```python
from build123d import *

# Parameters (mm, degrees)
SKETCH_2_W          = 9
SKETCH_2_H          = 6.5
EXTRUDE_1_DEPTH     = 90
SKETCH_3_R          = 3
CUT_EXTRUDE_1_DEPTH = 3.5
SKETCH_4_R          = 1.75
CUT_EXTRUDE_2_DEPTH = 91.346554998


with BuildPart() as part:
    # 草图2 → 凸台-拉伸1 (new body)
    with BuildSketch(Plane(origin=(0, 0, 0), x_dir=(0, 0, -1), z_dir=(1, 0, 0))):
        Rectangle(SKETCH_2_W, SKETCH_2_H)
    extrude(amount=EXTRUDE_1_DEPTH)

    # 草图3 → 切除-拉伸1 (cut)
    with BuildSketch(Plane(origin=(0, 3.25, 0), x_dir=(1, 0, 0), z_dir=(0, 1, 0))):
        with Locations(Location((15, 0, 0), (0, 0, 270))):
            Circle(SKETCH_3_R)
        with Locations(Location((35, 0, 0), (0, 0, 270))):
            Circle(SKETCH_3_R)
        with Locations(Location((55, 0, 0), (0, 0, 270))):
            Circle(SKETCH_3_R)
        with Locations(Location((75, 0, 0), (0, 0, 270))):
            Circle(SKETCH_3_R)
        with Locations((95, 0)):
            Circle(SKETCH_3_R)
        with Locations((115, 0)):
            Circle(SKETCH_3_R)
        with Locations((135, 0)):
            Circle(SKETCH_3_R)
        with Locations((155, 0)):
            Circle(SKETCH_3_R)
        with Locations((175, 0)):
            Circle(SKETCH_3_R)
        with Locations((195, 0)):
            Circle(SKETCH_3_R)
        with Locations((215, 0)):
            Circle(SKETCH_3_R)
        with Locations((235, 0)):
            Circle(SKETCH_3_R)
        with Locations((255, 0)):
            Circle(SKETCH_3_R)
    extrude(amount=-CUT_EXTRUDE_1_DEPTH, mode=Mode.SUBTRACT)

    # 草图4 → 切除-拉伸2 (cut, through all)
    with BuildSketch(Plane(origin=(0, 3.25, 0), x_dir=(1, 0, 0), z_dir=(0, 1, 0))):
        with Locations(Location((15, 0, 0), (0, 0, 270))):
            Circle(SKETCH_4_R)
        with Locations(Location((35, 0, 0), (0, 0, 270))):
            Circle(SKETCH_4_R)
        with Locations(Location((55, 0, 0), (0, 0, 270))):
            Circle(SKETCH_4_R)
        with Locations(Location((75, 0, 0), (0, 0, 270))):
            Circle(SKETCH_4_R)
        with Locations((95, 0)):
            Circle(SKETCH_4_R)
        with Locations((115, 0)):
            Circle(SKETCH_4_R)
        with Locations((135, 0)):
            Circle(SKETCH_4_R)
        with Locations((155, 0)):
            Circle(SKETCH_4_R)
        with Locations((175, 0)):
            Circle(SKETCH_4_R)
        with Locations((195, 0)):
            Circle(SKETCH_4_R)
        with Locations((215, 0)):
            Circle(SKETCH_4_R)
        with Locations((235, 0)):
            Circle(SKETCH_4_R)
        with Locations((255, 0)):
            Circle(SKETCH_4_R)
    extrude(amount=-CUT_EXTRUDE_2_DEPTH, mode=Mode.SUBTRACT)


solid = part.part
```
Geometry: final body of the model. Coordinates: model frame, mm. A direction names the side the tool comes from. Coordinates: 2 decimals unless noted, no trailing zeros. Order: outer loops, then holes, each group sorted by start corner. A loop starts at its lowest first (then second) coordinate and runs counter-clockwise, first axis right, second up. Notation, with made-up numbers: (37, 83) - (61, 83) arc R19 cw to (61, 112) - close; hole circle Ø10 at (-17.75, -11). An arc over 180 degrees is marked (long way). Write each question's results on one line, items separated by ' | '.
(1) Section query B-B, the plane x = 55. Return the cut outline in (y, z).
Values found:
outline: (-3.25, -4.5) - (3.25, -4.5) - (3.25, -3) - (-0.25, -3) - (-0.25, -1.75) - (-3.25, -1.75) - close; (-3.25, 1.75) - (-0.25, 1.75) - (-0.25, 3) - (3.25, 3) - (3.25, 4.5) - (-3.25, 4.5) - close
(2) First-contact query: pin 1 Ø3 at (x, z) = (76, 1) entering from +Y. Flat tip, straight axial feed; report the tip coordinate or a pass-through.
Values found:
pin 1: stops at y = -0.25
(3) Line query: line 1 (X direction, y = 0.65, z = 0); line 2 (X direction, y = -1, z = 0); line 3 (Z direction, x = 75, y = -1.5). Output: solid intervals per line, ascending. Write a range as [from, to].
Values found:
line 1: x = [0, 12], [18, 32], [38, 52], [58, 72], [78, 90] | line 2: x = [0, 13.25], [16.75, 33.25], [36.75, 53.25], [56.75, 73.25], [76.75, 90] | line 3: z = [-4.5, -1.75], [1.75, 4.5]
(4) Mould query, pull axis X, two halves, no side actions, for faces 1 (the face through (0, 0, 0)), 2 (the face through (33.29, -1.73, -0.38)), 3 (the face through (90, 0, 0)), 4 (the face through (44, 0, -4.5)). Classes: +X half, -X half, draft (parallel to the pull), parting line (faces both ways), or undercut.
Values found:
face 1: -X half | face 2: undercut | face 3: +X half | face 4: draft
(5) Set-up query: faces 5 (the face through (44, 0, 4.5)), 6 (the face through (33, -0.25, 0)). Return all of +Z, -Z, +X, -X, +Y, -Y with unobstructed straight access to the full face (end or side cutting, diameter ignored); none if empty.
Values found:
face 5: +Z, +X, -X, +Y, -Y | face 6: +Y
(6) Section query C-C, the plane z = 0. Count the separate pieces of the cut face and the enclosed holes in it, plus the area to 3 significant figures.
Values found:
separate pieces: 5 | enclosed holes: 0 | area: 459 mm²
(7) Section query A-A, the plane y = -1.5. Return the cut outline in (x, z), plus the area to 3 significant figures.
Values found:
outline: (0, -4.5) - (90, -4.5) - (90, 4.5) - (0, 4.5) - close; hole circle Ø3.5 at (15, 0); hole circle Ø3.5 at (35, 0); hole circle Ø3.5 at (55, 0); hole circle Ø3.5 at (75, 0) | area: 772 mm²
